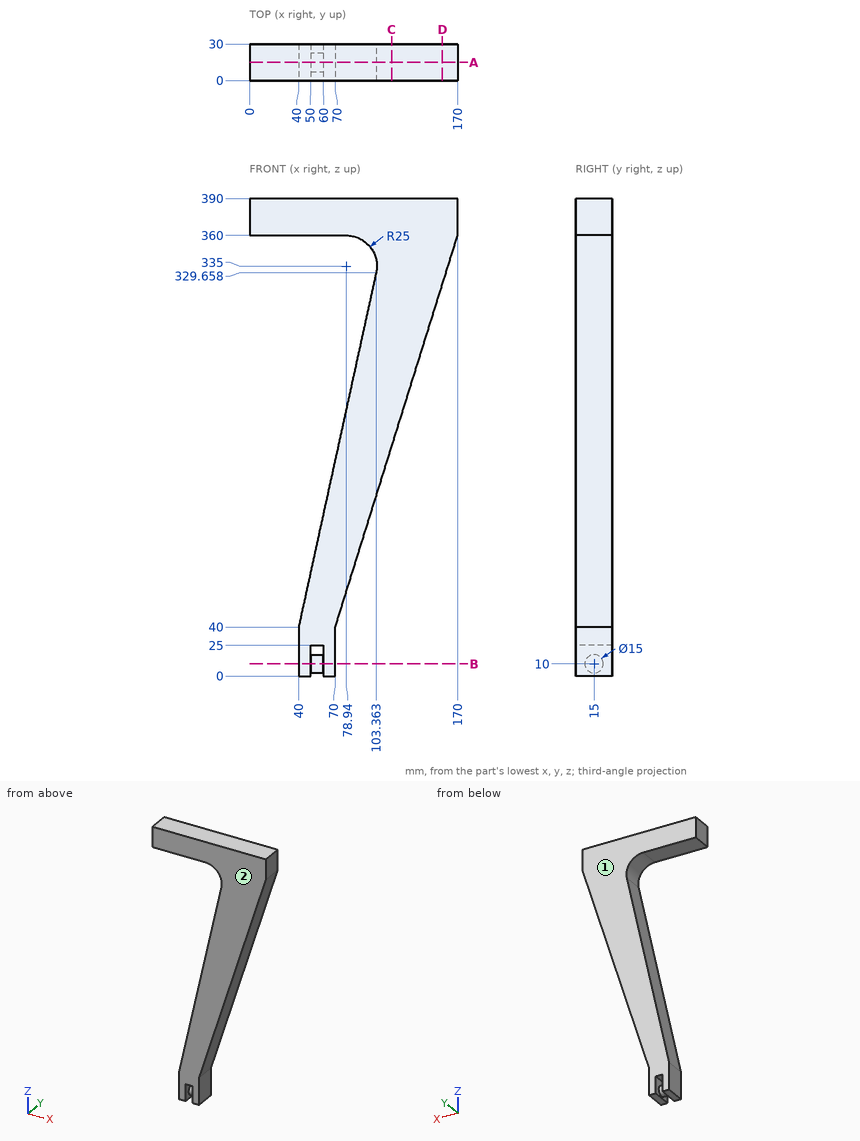
Study the drawing (mm; zero at the part's minimum x, y, z) and answer. Give positions to 0.01 mm unless a question says otherwise; leave off trailing zeros. Loops run counter-clockwise (first coordinate to the right, second up) from the corner with the lowest first, then second, coordinate; pieces in that order, holes last. Notation, with made-up numbers: (14, 40.25) - (24, 40.25) arc R22 cw to (24, 58.25) - close; hole circle Ø4 at (49.5, 81). An arc over 180 degrees is marked (long way). Return JSON: item names as keys, results as strings. Group by question number.
1. Determine the mould class of the marked faces 1 and 2 for opening direction Y: pulls with the +Y half, pulls with the -Y half, needs draft (parallel to the pull), parting line crosses it, or undercut.
2. Find section B-B (z = 10). Write down the section's boundary in (x, y), then the cut area to 3 significant figures.
3. Find section D-D (x = 157.5). Write down the section's boundary in (y, z).
4. Straight lines are drawn through the part: line 1 (Z direction, x = 18, y = 6); line 2 (X direction, y = 3, z = 97); line 3 (X direction, y = 27.25, z = 346) (1 decimal). For each, find the intervals that lie inside material, in ascending order. Write a range as [from, to].
5. Find section C-C (x = 116). Write down the section's boundary in (y, z).
6. Find section A-A (y = 15). Write down the section's boundary in (x, z), then the cut area to 3 significant figures.
7. Given pin 1 Ø1 at (y, z) = (14, 115) entering from -X; pin 2 Ø9 at (y, z) = (14, 28) entering from +X; pin 3 Ø3 at (y, z) = (5.5, 45) entering from -X (1 decimal); pin 4 Ø6 at (x, y) = (37.5, 7) entering from -Z, each flat-ended and moving along its own axis, determine where each tip first touches the part or whether it passes through.
Verdict:
{
 "1": {"face 1": "pulls with the +Y half", "face 2": "pulls with the -Y half"},
 "2": {"outline": "(40, 0) - (50, 0) - (50, 7.5) - (60, 7.5) - (60, 0) - (70, 0) - (70, 30) - (60, 30) - (60, 22.5) - (50, 22.5) - (50, 30) - (40, 30) - close", "area": "750 mm^2"},
 "3": {"outline": "(0, 320) - (30, 320) - (30, 390) - (0, 390) - close"},
 "4": {"line 1": "z = [360, 390]", "line 2": "x = [52.47, 87.81]", "line 3": "x = [101.4, 165.6]"},
 "5": {"outline": "(0, 187.2) - (30, 187.2) - (30, 390) - (0, 390) - close"},
 "6": {"outline": "(0, 360) - (78.94, 360) arc R25 cw to (103.36, 329.66) - (40, 40) - (40, 0) - (50, 0) - (50, 2.5) - (60, 2.5) - (60, 0) - (70, 0) - (70, 40) - (170, 360) - (170, 390) - (0, 390) - close; hole (50, 17.5) - (60, 17.5) - (60, 25) - (50, 25) - close", "area": "20,800 mm^2"},
 "7": {"pin 1": "stops at x = 56.3", "pin 2": "stops at x = 70", "pin 3": "stops at x = 40.8", "pin 4": "stops at z = 0"}
}
